Source: three-view drawing plus pictorial views. Frame: mm from the lowest corner of the part. A direction names the side the tool comes from. Give positions to 0.01 mm unless a question says otherwise; leave off trailing zeros. Order: outer loops, then holes, each group sorted by start corner. A loop starts at its lowest first (then second) coordinate and runs counter-clockwise, first axis right, second up.
1) Material intervals for line 1 (X direction, y = 4, z = 5.4); line 2 (X direction, y = 7.25, z = 3.6); line 3 (Z direction, x = 2.75, y = 3.5), sorted ascending.
2) First-contact query: P1, Ø0.6, axis at y = 4.5, z = 6, coming from the +X side; P2, Ø0.6, axis at y = 4.5, z = 6, coming from the -X side; P3, Ø0.6, axis at x = 3.5, z = 4.5, coming from the +Y side. Flat tips, straight axial feed; report the tip coordinate or a pass-through.
3) Section C-C, the plane z = 2. Return loops of the section in (x, y).
4) Draft query along Z for the marked faces 1, 2 and 3. Return one class per face: released by +Z, released by -Z, zero draft, split by the parting line, or undercut.
5) Section A-A, the plane y = 4. Return loops of the section in (x, z) (3 decimals).
6) Section B-B, the plane x = 8.25. Return loops of the section in (y, z), plus the area to 3 significant figures.
7) Section D-D, the plane x = 3. Return loops of the section in (y, z).
8) Access query for the marked faces 4, 5 and 6. Directions: +Z, -Z, +X, -X, +Y, -Y. A direction counts if a zero-diameter tool reaches every point of the face in a straight line with its end or side. Return the directions, or none.
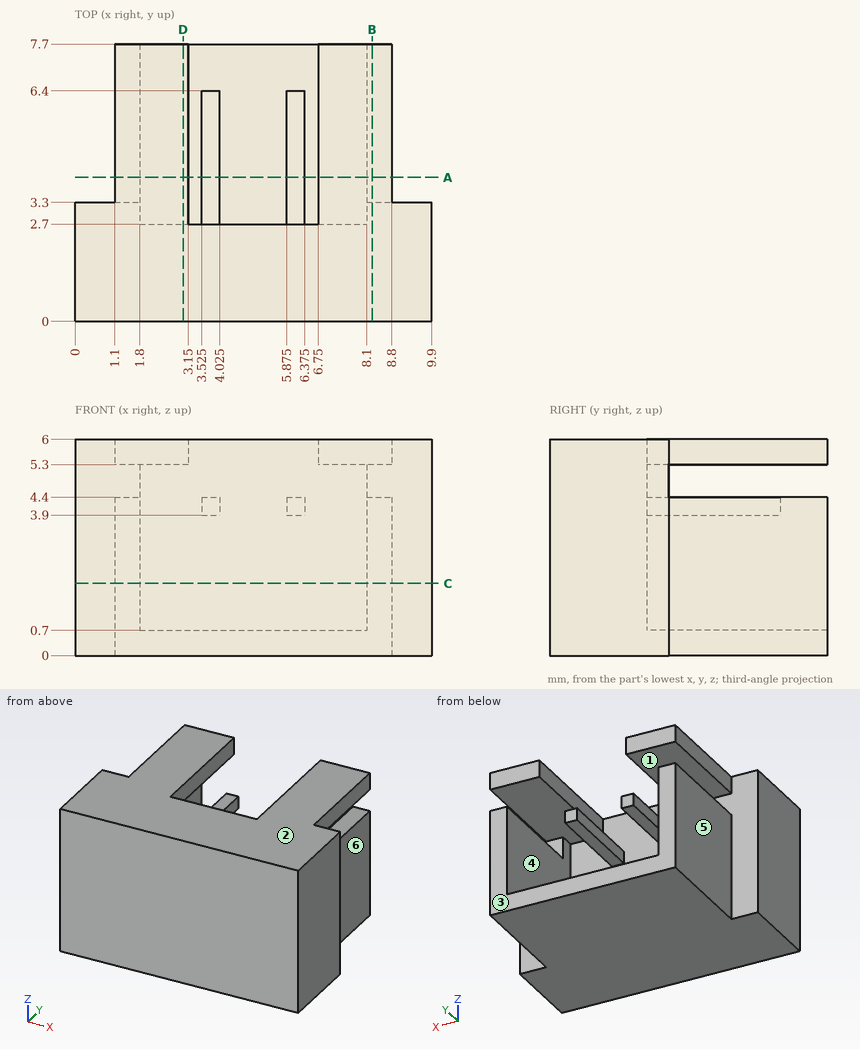
From the geometry:
1. line 1: x = 1.1 to 3.15, 6.75 to 8.8
1. line 2: x = 1.1 to 1.8, 8.1 to 8.8
1. line 3: z = 0 to 0.7, 5.3 to 6
2. P1: stops at x = 8.8
2. P2: stops at x = 1.1
2. P3: stops at y = 6.4
3. outline: (0, 0) - (9.9, 0) - (9.9, 3.3) - (8.8, 3.3) - (8.8, 7.7) - (8.1, 7.7) - (8.1, 2.7) - (1.8, 2.7) - (1.8, 7.7) - (1.1, 7.7) - (1.1, 3.3) - (0, 3.3) - close
4. face 1: undercut
4. face 2: released by +Z
4. face 3: zero draft
5. outline: (1.1, 0) - (8.8, 0) - (8.8, 4.4) - (8.1, 4.4) - (8.1, 0.7) - (1.8, 0.7) - (1.8, 4.4) - (1.1, 4.4) - close; (1.1, 5.3) - (3.15, 5.3) - (3.15, 6) - (1.1, 6) - close; (3.525, 3.9) - (4.025, 3.9) - (4.025, 4.4) - (3.525, 4.4) - close; (5.875, 3.9) - (6.375, 3.9) - (6.375, 4.4) - (5.875, 4.4) - close; (6.75, 5.3) - (8.8, 5.3) - (8.8, 6) - (6.75, 6) - close
6. outline: (0, 0) - (7.7, 0) - (7.7, 4.4) - (3.3, 4.4) - (3.3, 5.3) - (7.7, 5.3) - (7.7, 6) - (0, 6) - close
6. area: 42.2 mm2
7. outline: (0, 0) - (7.7, 0) - (7.7, 0.7) - (2.7, 0.7) - (2.7, 5.3) - (7.7, 5.3) - (7.7, 6) - (0, 6) - close
8. face 4: +Y
8. face 5: +Z, -Z, -X, +Y
8. face 6: +Z, -Z, +X, +Y
